The model under review builds one solid part; all positions refer to its coordinate system, in mm. A direction names the side the tool comes from. Coordinates: 2 decimals unless noted, no trailing zeros. Order: outer loops, then holes, each group sorted by start corner. A loop starts at its lowest first (then second) coordinate and runs counter-clockwise, first axis right, second up. Notation, with made-up numbers: (-24, 72.25) - (-18, 72.25) arc R7 cw to (-18, 85.25) - close; hole circle Ø8 at (0.25, 77). An arc over 180 degrees is marked (long way). Answer in a Markdown table with one row per item.
```python
from build123d import *

# Parameters (mm, degrees)
SKETCH_11_W         = 15
SKETCH_11_H         = 15
SKETCH_11_W_2       = 13
SKETCH_11_H_2       = 13
F_15X15X1_1_DEPTH   = 166
SKETCH_12_R         = 1.45
CUT_EXTRUDE_1_DEPTH = 85.677328725
SKETCH_13_R         = 1.45
CUT_EXTRUDE_2_DEPTH = 85.677328725


with BuildPart() as part:
    # 草图11 → 铝管 15X15X1(1) (new body)
    with BuildSketch(Plane(origin=(-83, 0, 0), x_dir=(0, 0, -1), z_dir=(1, 0, 0))):
        Rectangle(SKETCH_11_W, SKETCH_11_H)
        Rectangle(SKETCH_11_W_2, SKETCH_11_H_2, mode=Mode.SUBTRACT)
    extrude(amount=F_15X15X1_1_DEPTH)

    # 草图12 → 切除-拉伸1 (cut, through all)
    with BuildSketch(Plane(origin=(0, 0, -7.5), x_dir=(-1, 0, 0), z_dir=(0, 0, -1))):
        with Locations((-18.5, 0)):
            Circle(SKETCH_12_R)
        with Locations((18.5, 0)):
            Circle(SKETCH_12_R)
    extrude(amount=-CUT_EXTRUDE_1_DEPTH, mode=Mode.SUBTRACT)

    # 草图13 → 切除-拉伸2 (cut, through all)
    with BuildSketch(Plane.XZ.offset(7.5)):
        with Locations(Location((-77.5, 0, 0), (0, 0, 270))):
            Circle(SKETCH_13_R)
        with Locations(Location((-67.5, 0, 0), (0, 0, 270))):
            Circle(SKETCH_13_R)
        with Locations(Location((67.5, 0, 0), (0, 0, 270))):
            Circle(SKETCH_13_R)
        with Locations(Location((77.5, 0, 0), (0, 0, 270))):
            Circle(SKETCH_13_R)
    extrude(amount=-CUT_EXTRUDE_2_DEPTH, mode=Mode.SUBTRACT)


solid = part.part
```
Item 1: We need section A-A, the plane y = -5. Write out the cut boundary in (x, z).
Check values:
| item | result |
|---|---|
| outline | (-83, -7.5) - (83, -7.5) - (83, -6.5) - (-83, -6.5) - close; (-83, 6.5) - (83, 6.5) - (83, 7.5) - (-83, 7.5) - close |
Item 2: We need section B-B, the plane x = 67.5. Write out the cut boundary in (y, z), then the cut area to 3 significant figures.
Check values:
| item | result |
|---|---|
| outline | (-7.5, -7.5) - (7.5, -7.5) - (7.5, -1.45) - (6.5, -1.45) - (6.5, -6.5) - (-6.5, -6.5) - (-6.5, -1.45) - (-7.5, -1.45) - close; (-7.5, 1.45) - (-6.5, 1.45) - (-6.5, 6.5) - (6.5, 6.5) - (6.5, 1.45) - (7.5, 1.45) - (7.5, 7.5) - (-7.5, 7.5) - close |
| area | 50.2 mm^2 |
Item 3: To check wall thickness, follow line 1 (X direction, y = 6.8, z = 0); line 2 (Z direction, x = 27, y = -2.5). State the ranges of each line that lie inside material, in increasing order. Write a range as from..to.
Check values:
| item | result |
|---|---|
| line 1 | -83..-78.95, -76.05..-68.95, -66.05..66.05, 68.95..76.05, 78.95..83 |
| line 2 | -7.5..-6.5, 6.5..7.5 |
Item 4: Mouldability with a two-part tool opening along Y and no side actions: class faces 1 (the face through (-1, -7.5, 0)), 2 (the face through (76.084, -7.007, 0.314)), 3 (the face through (-1, 6.5, 0)) as +Y half, -Y half, draft (parallel to the pull), parting line (faces both ways), or undercut.
Check values:
| item | result |
|---|---|
| face 1 | -Y half |
| face 2 | draft |
| face 3 | undercut |
Item 5: Tool access review of faces 4 (the face through (-1, -6.5, 0)), 5 (the face through (17.12, 0.44, -7.01)): name each direction out of +Z, -Z, +X, -X, +Y, -Y from which nothing blocks a thin tool from reaching the whole face with its end or side.
Check values:
| item | result |
|---|---|
| face 4 | +X, -X |
| face 5 | +Z, -Z |
Item 6: We need section C-C, the plane x = 47. Write out the cut boundary in (y, z), then the cut area to 3 significant figures.
Check values:
| item | result |
|---|---|
| outline | (-7.5, -7.5) - (7.5, -7.5) - (7.5, 7.5) - (-7.5, 7.5) - close; hole (-6.5, -6.5) - (6.5, -6.5) - (6.5, 6.5) - (-6.5, 6.5) - close |
| area | 56.0 mm^2 |
Item 7: We need section D-D, the plane z = 0. State how many separate pieces and enclosed holes the cut face has, then the cut area to 3 significant figures.
Check values:
| item | result |
|---|---|
| separate pieces | 10 |
| enclosed holes | 0 |
| area | 309 mm^2 |
